Autodesk Inventor part; units mm, degrees
ref_plane "YZ Plane" through (0, 0, 0) normal (1, 0, 0) x (0, 1, 0)
ref_plane "XZ Plane" through (0, 0, 0) normal (0, 1, 0) x (-1, 0, 0)
ref_plane "XY Plane" through (0, 0, 0) normal (0, 0, 1) x (1, 0, 0)
sketch "Szkic1" plane through (0, 0, 0) normal (0, 1, 0) x (-1, 0, 0)
  circle A0 centre (0, 0) radius 20
  circle A1 centre (0, 0) radius 26.5
  line L0 (0, 26.5) -> (0, 20)
  circle A2 centre (0, 23.25) radius 1.6
  circle A3 centre (-16.4402, 16.4402) radius 1.6
  circle A4 centre (-23.25, 0) radius 1.6
  circle A5 centre (-16.4402, -16.4402) radius 1.6
  circle A6 centre (0, -23.25) radius 1.6
  circle A7 centre (16.4402, -16.4402) radius 1.6
  circle A8 centre (23.25, 0) radius 1.6
  circle A9 centre (16.4402, 16.4402) radius 1.6
  dimension "d0" = 40
  dimension "d1" = 53
  dimension "d2" = 3.2
  dimension "d5" = 360
extrude "Wyciągnięcie proste1" add sketch "Szkic1" along normal blind 2 contours A0 | A1
sketch "Szkic3" plane through (0, 2, 0) normal (0, 1, 0) x (1, 0, 0)
  circle A0 centre (0, 0) radius 5
  circle A1 centre (5, 0) radius 1.65
  circle A2 centre (-2.5, 4.3301) radius 1.65
  circle A3 centre (-2.5, -4.3301) radius 1.65
  point P0 (1.5451, -4.7553)
  point P1 (1.5451, 4.7553)
  point P2 (-4.0451, 2.9389)
  dimension "d22" = 10
  dimension "d39" = 3.3
  dimension "d42" = 360
hole "Otwór2" at (5, 2, 0) at (-2.5, 2, -4.3301) at (-2.5, 2, 4.3301) direction (0, -1, 0) diameter 3.3 end through all
properties part number "Bell_KoloFormaDol"
Work out the finished part from the listing and answer in its coordinate system (mm). Give positions to 0.01 mm unless a question says otherwise; leave off trailing zeros. Write each loop counter-clockwise with the first axis right and the second up, starting at its lowest first coordinate (ties: lowest second). Pieces come first, ordered by that corner, then holes.
Q1. Straight lines are drawn through the part: L1, parallel to Z at x = -3, y = 1.75; L2, parallel to Z at x = 15, y = 0.2; L3, parallel to Z at x = 6.5, y = 0.65. For each, find the intervals that lie inside material, in ascending order.
Answer:
L1: z = -26.33 to -5.9, -2.76 to 2.76, 5.9 to 26.33
L2: z = -21.85 to -17.14, -15.74 to 15.74, 17.14 to 21.85
L3: z = -25.69 to -0.69, 0.69 to 25.69
Q2. The part is cut by section A-A on z = 0. Give the vertices of the cut face in (x, y), and give its area (3 significant figures).
Answer:
outline: (-26.5, 0) - (-24.85, 0) - (-24.85, 2) - (-26.5, 2) - close; (-21.65, 0) - (3.35, 0) - (3.35, 2) - (-21.65, 2) - close; (6.65, 0) - (21.65, 0) - (21.65, 2) - (6.65, 2) - close; (24.85, 0) - (26.5, 0) - (26.5, 2) - (24.85, 2) - close
area: 86.6 mm2
Q3. The part is cut by section C-C on x = 23.25. Give the vertices of the cut face in (y, z), and give its area (3 significant figures).
Answer:
outline: (0, -12.72) - (2, -12.72) - (2, -1.6) - (0, -1.6) - close; (0, 1.6) - (2, 1.6) - (2, 12.72) - (0, 12.72) - close
area: 44.5 mm2
Q4. The part is cut by section B-B on x = 0. Give the vertices of the cut face in (y, z), and give its area (3 significant figures).
Answer:
outline: (0, -26.5) - (2, -26.5) - (2, -24.85) - (0, -24.85) - close; (0, -21.65) - (2, -21.65) - (2, 21.65) - (0, 21.65) - close; (0, 24.85) - (2, 24.85) - (2, 26.5) - (0, 26.5) - close
area: 93.2 mm2
Q5. The part is cut by section D-D on z = 23.25. Give the vertices of the cut face in (x, y).
Answer:
outline: (-12.72, 0) - (-1.6, 0) - (-1.6, 2) - (-12.72, 2) - close; (1.6, 0) - (12.72, 0) - (12.72, 2) - (1.6, 2) - close
Q6. Given pin 1 (1 mm diameter, centred on x = 4.5, y = 1, fed in from +Z), flat-ended and moving along its own axis, determine where the tip first touches the part or whether it passes through.
Answer:
pin 1: stops at z = 26.2
Q7. For a pull along Z with two mould halves and no side action, classify faces 1 (the face through (0, 0, 0)), 2 (the face through (-14.246, 0.986, -22.345)), 3 (the face through (-16.232, 0.986, -18.027)), 4 (the face through (17.62, 0.99, -17.52)) as released by +Z, released by -Z, zero draft, split by the parting line, or undercut.
Answer:
face 1: zero draft
face 2: split by the parting line
face 3: undercut
face 4: undercut
